Check sheet for the modelled part. Datum: model origin and axes. Units: mm. Face numbers are marked on the shaded views. A direction names the side the tool comes from. Round coordinates to 2 decimals unless told otherwise and drop trailing zeros. Write each loop counter-clockwise with the first axis right and the second up, starting at its lowest first coordinate (ties: lowest second). Pieces come first, ordered by that corner, then holes. Notation, with made-up numbers: (60, 16.5) -> (81, 16.5) arc R28 cw to (81, 50.5) -> close; hole circle Ø11 at (14.25, -36.75). An arc over 180 degrees is marked (long way). Write item = value, one per line.
from build123d import *

# Parameters (mm, degrees)
ESQUISSE2_W             = 44
ESQUISSE2_H             = 44
BOSS_EXTRU_1_DEPTH      = 10
ESQUISSE3_W             = 36
ESQUISSE3_H             = 36
BOSS_EXTRU_2_DEPTH      = 10
ESQUISSE4_W             = 42.5
ESQUISSE4_H             = 42.5
ESQUISSE4_W_2           = 36
ESQUISSE4_H_2           = 36
ENL_V_MAT_EXTRU_1_DEPTH = 5
CONG_1_R                = 3
CONG_2_R                = 2
BOSS_EXTRU_4_DEPTH      = 1


with BuildPart() as part:
    # Esquisse2 → Boss.-Extru.1 (new body)
    with BuildSketch(Plane.XY):
        with Locations((22, 22)):
            Rectangle(ESQUISSE2_W, ESQUISSE2_H)
    extrude(amount=BOSS_EXTRU_1_DEPTH)

    # Esquisse3 → Boss.-Extru.2 (add)
    with BuildSketch(Plane(origin=(0, 0, 0), x_dir=(-1, 0, 0), z_dir=(0, 0, -1))):
        with Locations((-22, 22)):
            Rectangle(ESQUISSE3_W, ESQUISSE3_H)
    extrude(amount=BOSS_EXTRU_2_DEPTH)

    # Esquisse4 → Enlèv. mat.-Extru.1 (cut)
    with BuildSketch(Plane(origin=(0, 0, 0), x_dir=(-1, 0, 0), z_dir=(0, 0, -1))):
        with Locations((-22.75, 21.25)):
            Rectangle(ESQUISSE4_W, ESQUISSE4_H)
        with Locations((-22, 22)):
            Rectangle(ESQUISSE4_W_2, ESQUISSE4_H_2, mode=Mode.SUBTRACT)
    extrude(amount=-ENL_V_MAT_EXTRU_1_DEPTH, mode=Mode.SUBTRACT)

    # Congé1
    cong_1_edges = [part.edges().sort_by_distance(p)[0] for p in [
        (22, 40, -10),
        (4, 22, -10),
        (22, 4, -10),
        (40, 22, -10),
        (44, 0, 7.5),
        (44, 44, 5),
        (0, 0, 5),
        (0, 44, 5),
        (1.5, 42.5, 2.5),
        (4, 4, -2.5),
        (4, 40, -2.5),
        (40, 4, -2.5),
        (40, 40, -2.5),
    ]]
    fillet(cong_1_edges, radius=CONG_1_R)

    # Congé2
    cong_2_edges = [part.edges().sort_by_distance(p)[0] for p in [
        (44, 22, 10),
        (22, 0, 10),
        (0, 22, 10),
        (22, 44, 10),
        (0.878679656, 43.121320344, 10),
        (0.878679656, 0.878679656, 10),
        (43.121320344, 43.121320344, 10),
        (43.121320344, 0.878679656, 10),
    ]]
    fillet(cong_2_edges, radius=CONG_2_R)

    # Esquisse7 → Boss.-Extru.4 (add)
    with BuildSketch(Plane.XY.offset(10)):
        with BuildLine():
            Line((15.374098957, 17.346843443), (18.030348957, 14.221843443))
            add(Edge.make_bspline(
                [(18.030348957, 14.221843443), (17.301182291, 14.32601011), (16.565114838, 14.389890267), (15.842848957, 14.534343443), (15.423010802, 14.618311074), (14.838115665, 15.028795794), (14.436598957, 15.315593443), (12.049681404, 17.020534553), (11.595795075, 19.293760446), (11.936598957, 22.190593443), (12.054157826, 23.189843826), (13.69238751, 25.196381996), (14.436598957, 25.940593443)],
                knots=[0, 0, 0, 0, 1, 1, 1, 2, 2, 2, 3, 3, 3, 4, 4, 4, 4], degree=3))
            Line((14.436598957, 25.940593443), (15.06939707, 26.573391556))
            Line((15.06939707, 26.573391556), (14.905348957, 25.784343443))
            add(Edge.make_bspline(
                [(14.905348957, 25.784343443), (14.590446041, 23.265120116), (14.091309116, 20.570212966), (14.905348957, 18.128093443), (15.001385879, 17.839982679), (15.278062036, 17.634954207), (15.374098957, 17.346843443)],
                knots=[0, 0, 0, 0, 1, 1, 1, 2, 2, 2, 2], degree=3))
        make_face()
        with BuildLine():
            Line((30.686598957, 11.878093443), (26.780348957, 10.784343443))
            Line((26.780348957, 10.784343443), (20.999098957, 11.878093443))
            Line((20.999098957, 11.878093443), (29.124098957, 13.909343443))
            ThreePointArc((29.124098957, 13.909343443), (30.444920086, 13.308773157), (30.686598957, 11.878093443))
        make_face()
        with BuildLine():
            Line((18.811598957, 7.971843443), (14.280348957, 5.471843443))
            add(Edge.make_bspline(
                [(14.280348957, 5.471843443), (14.280348957, 7.772797666), (14.593726557, 7.189715843), (13.342848957, 8.440593443)],
                knots=[0, 0, 0, 0, 1, 1, 1, 1], degree=3))
            add(Edge.make_bspline(
                [(13.342848957, 8.440593443), (13.394932291, 8.54476011), (13.404330032, 8.685401354), (13.499098957, 8.753093443), (13.783405732, 8.956169711), (14.089133052, 9.185268084), (14.436598957, 9.221843443), (16.134694919, 9.400590386), (17.384797269, 8.685244287), (18.811598957, 7.971843443)],
                knots=[0, 0, 0, 0, 1, 1, 1, 2, 2, 2, 3, 3, 3, 3], degree=3))
        make_face()
        with BuildLine():
            Line((13.200641117, 12.506283222), (29.317230938, 9.618393711))
            ThreePointArc((29.317230938, 9.618393711), (28.067553161, 8.724486443), (28.200641117, 7.193783222))
            Line((28.200641117, 7.193783222), (12.575641117, 10.631283222))
            ThreePointArc((12.575641117, 10.631283222), (12.499815902, 11.698224961), (13.200641117, 12.506283222))
        make_face()
        with BuildLine():
            add(Edge.make_bspline(
                [(20.999098957, 15.315593443), (20.827145061, 14.799731755), (21.046210645, 13.925047339), (20.530348957, 13.753093443), (20.153128088, 13.627353153), (20.137873233, 14.301819167), (20.061598957, 14.378093443), (16.567694762, 17.871997638), (14.613515541, 21.933204334), (16.467848957, 26.878093443), (17.971713728, 30.888399498), (21.846423142, 33.698659479), (22.249098957, 38.128093443)],
                knots=[4, 4, 4, 4, 5, 5, 5, 6, 6, 6, 7, 7, 7, 8, 8, 8, 8], degree=3))
            add(Edge.make_bspline(
                [(22.249098957, 38.128093443), (23.024720103, 37.74028287), (26.549972992, 30.317022339), (26.624098957, 29.378093443), (26.824723104, 26.836854256), (26.793735434, 25.141457588), (26.311598957, 22.971843443), (25.843661476, 20.866124777), (23.763276375, 19.341691827), (22.561598957, 17.659343443), (22.093633816, 17.004192245), (21.257183639, 16.089847489), (20.999098957, 15.315593443)],
                knots=[0, 0, 0, 0, 1, 1, 1, 2, 2, 2, 3, 3, 3, 4, 4, 4, 4], degree=3))
        make_face()
        with BuildLine():
            add(Edge.make_bspline(
                [(22.874098957, 14.378093443), (22.776875457, 14.340699789), (22.561598957, 14.273926776), (22.561598957, 14.378093443), (22.561598957, 17.724570677), (25.385181625, 19.244008778), (26.780348957, 22.034343443), (28.269529967, 25.012705463), (27.627114524, 26.898375507), (27.405348957, 30.003093443)],
                knots=[3, 3, 3, 3, 4, 4, 4, 5, 5, 5, 6, 6, 6, 6], degree=3))
            add(Edge.make_bspline(
                [(27.405348957, 30.003093443), (30.439237099, 28.486149372), (31.410808057, 20.585108609), (29.749098957, 17.815593443), (28.578255605, 15.864187855), (26.718288261, 15.58655694), (24.749098957, 15.003093443), (24.117435238, 14.815933822), (23.488994366, 14.614591677), (22.874098957, 14.378093443)],
                knots=[0, 0, 0, 0, 1, 1, 1, 2, 2, 2, 3, 3, 3, 3], degree=3))
        make_face()
        with BuildLine():
            add(Edge.make_bspline(
                [(13.825641117, 6.383595142), (13.664946359, 4.294397314), (12.835062605, 4.491118619), (11.307669526, 4.983380758)],
                knots=[1, 1, 1, 1, 2, 2, 2, 2], degree=3))
            add(Edge.make_bspline(
                [(11.307669526, 4.983380758), (10.888236852, 8.443524348), (13.995704046, 8.594588879), (13.825641117, 6.383595142)],
                knots=[0, 0, 0, 0, 1, 1, 1, 1], degree=3))
        make_face()
        with BuildLine():
            add(Edge.make_bspline(
                [(30.312986898, 9.093826211), (32.34922339, 8.599547626), (32.02172038, 7.812052803), (31.290447284, 6.383595142)],
                knots=[1, 1, 1, 1, 2, 2, 2, 2], degree=3))
            add(Edge.make_bspline(
                [(31.290447284, 6.383595142), (27.807867011, 6.525553152), (28.158042034, 9.616920214), (30.312986898, 9.093826211)],
                knots=[0, 0, 0, 0, 1, 1, 1, 1], degree=3))
        make_face()
    extrude(amount=BOSS_EXTRU_4_DEPTH)


solid = part.part
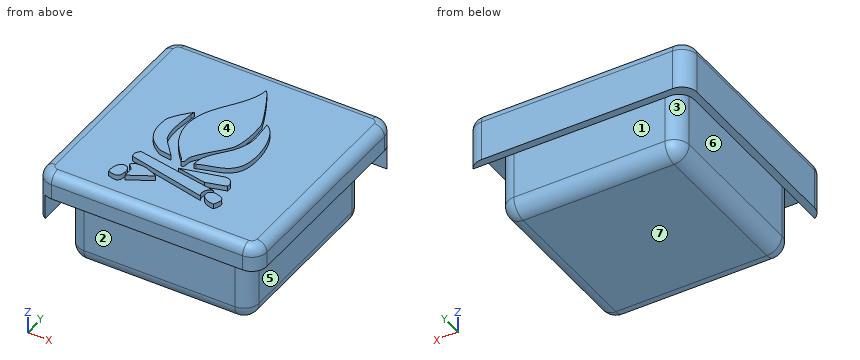
(1) Access from +Z, -Z, +X, -X, +Y, -Y to the whole of each face (thin tool, end or side, straight path). Record for the marked faces 1, 2, 3 and 4.
Worked answers:
face_1 = -Z, +X
face_2 = -Z, +X, -Y
face_3 = -Z
face_4 = +Z, +X, -X, +Y, -Y
(2) Material ranges on L1, parallel to X at y = 26.5, z = 4.5; L2, parallel to Z at x = 7, y = 17; L3, parallel to X at y = 12.5, z = -4.5, recorded low to high. Write a range as [from, to].
Worked answers:
L1 = [0, 1.5], [4, 40]
L2 = [-10, 10]
L3 = [4, 40]
(3) Sectioned sample at C-C on z = -4.5. Enter the section's corners in (x, y), then the cut area to 3 significant figures.
Worked answers:
outline = (4, 7) arc R3 ccw to (7, 4) -> (37, 4) arc R3 ccw to (40, 7) -> (40, 37) arc R3 ccw to (37, 40) -> (7, 40) arc R3 ccw to (4, 37) -> close
area = 1,290 mm²
(4) Go/stop test with flat-tipped pins: P1, Ø1.5, axis at x = 17.5, z = 2, coming from the -Y side; P2, Ø1.5, axis at y = 22, z = 3.5, coming from the +X side; P3, Ø8, axis at y = 28.5, z = -6.5, coming from the -X side. Record where each tip stops, or that it passes through.
Worked answers:
P1 = 4
P2 = 40
P3 = 4
(5) Sectioned sample at D-D on x = 6. Enter the section's corners in (y, z).
Worked answers:
outline = (0, 5) -> (4.17, 5) -> (4.17, -7) arc R2.83 ccw to (7, -9.83) -> (37, -9.83) arc R2.83 ccw to (39.83, -7) -> (39.83, 5) -> (42.5, 5) -> (42.5, 0) -> (44, 0) -> (44, 8) arc R2 ccw to (42, 10) -> (2, 10) arc R2 ccw to (0, 8) -> close
(6) Release check for a two-part mould opening along X. For the marked faces 5, 6 and 7 record: pulls with the +X half, pulls with the -X half, needs draft (parallel to the pull), parting line crosses it, or undercut.
Worked answers:
face_5 = pulls with the +X half
face_6 = undercut
face_7 = needs draft
(7) Sectioned sample at B-B on x = 34. Enter the section's corners in (y, z), then the cut area to 3 significant figures.
Worked answers:
outline = (0, 5) -> (4, 5) -> (4, -7) arc R3 ccw to (7, -10) -> (37, -10) arc R3 ccw to (40, -7) -> (40, 5) -> (42.5, 5) -> (42.5, 0) -> (44, 0) -> (44, 8) arc R2 ccw to (42, 10) -> (2, 10) arc R2 ccw to (0, 8) -> close
area = 762 mm²
(8) Sectioned sample at A-A on z = 2.5. Enter the section's corners in (x, y), then the cut area to 3 significant figures.
Worked answers:
outline = (0, 3) arc R3 ccw to (1.5, 0.4) -> (1.5, 39.5) arc R3 cw to (4.5, 42.5) -> (43.6, 42.5) arc R3 ccw to (41, 44) -> (3, 44) arc R3 ccw to (0, 41) -> close; (4, 7) arc R3 ccw to (7, 4) -> (37, 4) arc R3 ccw to (40, 7) -> (40, 37) arc R3 ccw to (37, 40) -> (7, 40) arc R3 ccw to (4, 37) -> close
area = 1,410 mm²
